Can you work these out from the model? Positions are in its coordinate system, mm. Coordinates: 2 decimals unless noted, no trailing zeros. Order: outer loops, then holes, each group sorted by start corner. A loop starts at its lowest first (then second) coordinate and runs counter-clockwise, first axis right, second up. Notation, with made-up numbers: (-30.75, 28.5) -> (-2.75, 28.5) arc R24 ccw to (-2.75, 66.5) -> close; hole circle Ø9 at (67.5, 67.5). An arc over 180 degrees is marked (long way). Answer as a JSON object with one key per item and string values. Group by question number.
(1) For pin 1 (6.5 mm diameter, centred on x = 0, z = 0, fed in from +Y), with a flat end and sliding along its axis, tell me the tip position at first contact or that it passes through.
(2) If we mould it in two halves opening along Z, with no side actions, what happens to faces 1 (the flat face through (-2, 0, -14)), 2 (the cylindrical face through (0.867, -0.373, 3.905))? For each: pulls with the +Z half, pulls with the -Z half, needs draft (parallel to the pull), parting line crosses it, or undercut.
(3) I want a section at A-A, the plane z = 0. List the corners of the cut face in (x, y) for me, plus the area to 3 significant figures.
(4) I want a section at B-B, the plane x = 0. List the corners of the cut face in (y, z) for me, plus the area to 3 significant figures.
(5) I need wall thicknesses on line 1 (Z direction, x = 0, y = -0.4); line 2 (X direction, y = -0.2, z = -1). Which ranges of each line are inside material? Lowest first, please.
from build123d import *

# Parameters (mm, degrees)
SKETCH1_W                = 240
SKETCH1_H                = 120
BASE_FLANGE1_DEPTH       = 0.7366
F_4_0_4_DIAMETER_HOLE1_D = 8


# Sheet-metal steps are written as plain solids
with BuildPart() as part:
    # Sketch1 → Base-Flange1 (new body)
    with BuildSketch(Plane(origin=(0, 0, 0), x_dir=(1, 0, 0), z_dir=(0, 1, 0))):
        Rectangle(SKETCH1_W, SKETCH1_H)
    extrude(amount=-BASE_FLANGE1_DEPTH)

    # Ø4.0 (4) Diameter Hole1 (through all)
    with Locations(Plane(origin=(0, 0, 0), x_dir=(1, 0, 0), z_dir=(0, 1, 0))):
        with Locations((0, 0)):
            Hole(F_4_0_4_DIAMETER_HOLE1_D / 2)


solid = part.part
Computed values:
{
 "1": {"pin 1": "passes through"},
 "2": {"face 1": "needs draft", "face 2": "undercut"},
 "3": {"outline": "(-120, -0.74) -> (-4, -0.74) -> (-4, 0) -> (-120, 0) -> close; (4, -0.74) -> (120, -0.74) -> (120, 0) -> (4, 0) -> close", "area": "171 mm2"},
 "4": {"outline": "(-0.74, -60) -> (0, -60) -> (0, -4) -> (-0.74, -4) -> close; (-0.74, 4) -> (0, 4) -> (0, 60) -> (-0.74, 60) -> close", "area": "82.5 mm2"},
 "5": {"line 1": "z = -60 to -4, 4 to 60", "line 2": "x = -120 to -3.87, 3.87 to 120"}
}
